```python
from build123d import *

# Parameters (mm, degrees)
F0_W     = 482.6
F0_H     = 419.1
F1_DEPTH = 152.4
F2_W     = 438.15
F2_H     = 260.35
F3_DEPTH = 241.3


with BuildPart() as f1:
    # F0 (on Front) → F1 (new body, symmetric)
    with BuildSketch(Plane.XZ):
        Rectangle(F0_W, F0_H)
    extrude(amount=F1_DEPTH, both=True)

    # F2 (on face) → F3 (cut, symmetric)
    with BuildSketch(Plane.XY.offset(209.55)):
        Rectangle(F2_W, F2_H)
    extrude(amount=F3_DEPTH, both=True, mode=Mode.SUBTRACT)


solid = f1.part
```
Verification items for the finished model (mm, model axes). A direction names the side the tool comes from. Give positions to 0.01 mm unless a question says otherwise; leave off trailing zeros. Write each loop counter-clockwise with the first axis right and the second up, starting at its lowest first coordinate (ties: lowest second). Pieces come first, ordered by that corner, then holes. Notation, with made-up numbers: M 63.5,-32.5 L 92.5,-32.5 A28 cw 92.5,-14.5 Z; hole C 75,-9 d7. An arc over 180 degrees is marked long. One line per question, with ' | ' between items.
1) Mould release check, pull along X, two halves, no side actions. Record for faces 3 (the flat face through (-3, 2, -31.75)), 4 (the flat face through (241.3, -2, -3)), 5 (the flat face through (-241.3, -2, -3)): released by +X, released by -X, zero draft, split by the parting line, or undercut.
Result:
face 3: undercut | face 4: released by +X | face 5: released by -X
2) Set-up check for faces 1 (the flat face through (-3, -152.4, 3)), 2 (the flat face through (219.075, -2, 91)): record each of +Z, -Z, +X, -X, +Y, -Y from which the full face is reachable in a straight line by a thin tool's end or side.
Result:
face 1: +Z, -Z, +X, -X, -Y | face 2: +Z
3) Section check B-B on y = -124.5. Enter the section's corners in (x, z) (3 decimals), plus the area to 3 significant figures.
Result:
outline: M -241.3,-209.55 L 241.3,-209.55 L 241.3,209.55 L 219.075,209.55 L 219.075,-31.75 L -219.075,-31.75 L -219.075,209.55 L -241.3,209.55 Z | area: 96,500 mm2
4) Section check C-C on x = -173. Enter the section's corners in (y, z) (3 decimals), plus the area to 3 significant figures.
Result:
outline: M -152.4,-209.55 L 152.4,-209.55 L 152.4,209.55 L 130.175,209.55 L 130.175,-31.75 L -130.175,-31.75 L -130.175,209.55 L -152.4,209.55 Z | area: 64,900 mm2
5) Section check A-A on z = 166. Enter the section's corners in (x, y) (3 decimals), plus the area to 3 significant figures.
Result:
outline: M -241.3,-152.4 L 241.3,-152.4 L 241.3,152.4 L -241.3,152.4 Z; hole M -219.075,-130.175 L 219.075,-130.175 L 219.075,130.175 L -219.075,130.175 Z | area: 33,000 mm2
6) Gauge pin test, flat end, axial feed: pin 1 Ø1.5 at (x, y) = (136.5, -15) entering from +Z. Record the tip position at first contact, or that the pin passes through.
Result:
pin 1: stops at z = -31.75
7) Thickness scan on line 1 along Y through (x, z) = (-126.5, 106) (3 decimals); line 2 along X through (y, z) = (110, 18.5) (3 decimals); line 3 along Z through (x, y) = (9.5, -67). Record the ranges inside material, lowest first. Write a range as [from, to].
Result:
line 1: y = [-152.4, -130.175], [130.175, 152.4] | line 2: x = [-241.3, -219.075], [219.075, 241.3] | line 3: z = [-209.55, -31.75]
